```python
from build123d import *

# Parameters (mm, degrees)
BOSS_EXTRU_1_DEPTH      = 1
ESQUISSE2_R             = 1.5
ESQUISSE2_R_2           = 0.5
ENL_V_MAT_EXTRU_1_DEPTH = 18


with BuildPart() as part:
    # Esquisse1 → Boss.-Extru.1 (new body)
    with BuildSketch(Plane.XY):
        with BuildLine():
            Line((-4, 2.530340064), (-4, 15.530340064))
            ThreePointArc((-4, 15.530340064), (0, 19.530340064), (4, 15.530340064))
            Line((4, 15.530340064), (4, 2.530340064))
            Line((4, 2.530340064), (16.535533906, 2.530340064))
            ThreePointArc((16.535533906, 2.530340064), (20.535533906, -1.469659936), (16.535533906, -5.469659936))
            Line((16.535533906, -5.469659936), (4, -5.469659936))
            Line((4, -5.469659936), (4, -19.398592124))
            ThreePointArc((4, -19.398592124), (0, -23.398592124), (-4, -19.398592124))
            Line((-4, -19.398592124), (-4, -5.469659936))
            Line((-4, -5.469659936), (-17.464466094, -5.469659936))
            ThreePointArc((-17.464466094, -5.469659936), (-21.464466094, -1.469659936), (-17.464466094, 2.530340064))
            Line((-17.464466094, 2.530340064), (-4, 2.530340064))
        make_face()
    extrude(amount=BOSS_EXTRU_1_DEPTH)

    # Esquisse2 → Enlèv. mat.-Extru.1 (cut)
    with BuildSketch(Plane.XY.offset(1)):
        with Locations((0, 15.030340064)):
            Circle(ESQUISSE2_R)
        with Locations((16.5, -1.469659936)):
            Circle(ESQUISSE2_R)
        with Locations((0, -17.969659936)):
            Circle(ESQUISSE2_R)
        with Locations((-16.5, -1.469659936)):
            Circle(ESQUISSE2_R)
        with Locations((0, -1.469659936)):
            Circle(ESQUISSE2_R_2)
    extrude(amount=-ENL_V_MAT_EXTRU_1_DEPTH, mode=Mode.SUBTRACT)


solid = part.part
```
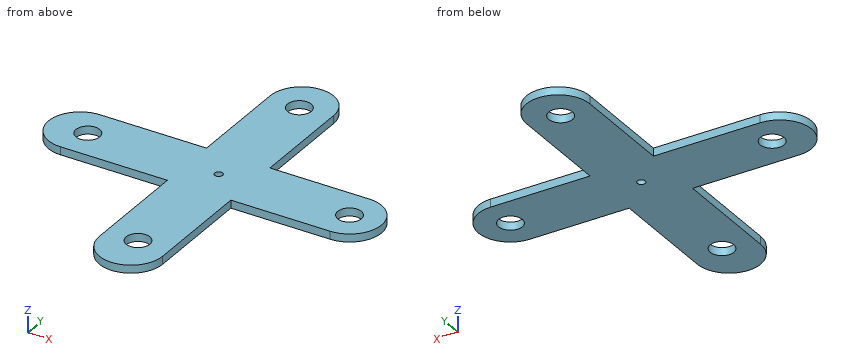
The listing builds one solid part. Answer for the finished solid, in the listing's coordinates (mm). Round coordinates to 2 decimals unless told otherwise and drop trailing zeros. Loops run counter-clockwise (first coordinate to the right, second up) from the corner with the lowest first, then second, coordinate; pieces in that order, holes last.
1) A cutting plane is placed at A-A on x = 0. Determine the outline of the cut face in (y, z).
Outcome:
outline: (-23.4, 0) - (-19.47, 0) - (-19.47, 1) - (-23.4, 1) - close; (-16.47, 0) - (-1.97, 0) - (-1.97, 1) - (-16.47, 1) - close; (-0.97, 0) - (13.53, 0) - (13.53, 1) - (-0.97, 1) - close; (16.53, 0) - (19.53, 0) - (19.53, 1) - (16.53, 1) - close
2) A cutting plane is placed at B-B on x = -16.5. Determine the outline of the cut face in (y, z).
Outcome:
outline: (-5.47, 0) - (-2.97, 0) - (-2.97, 1) - (-5.47, 1) - close; (0.03, 0) - (2.53, 0) - (2.53, 1) - (0.03, 1) - close
3) Given P1, Ø0.5, axis at x = -10, z = 0.5, coming from the -Y side; P2, Ø0.5, axis at x = 9.5, z = 0.5, coming from the +Y side, each flat-ended and moving along its own axis, determine where each tip first touches the part or whether it passes through.
Outcome:
P1: stops at y = -5.47
P2: stops at y = 2.53
4) A cutting plane is placed at D-D on z = 0.4. Determine the outline of the cut face in (x, y).
Outcome:
outline: (-17.46, -5.47) - (-4, -5.47) - (-4, -19.4) arc R4 ccw to (4, -19.4) - (4, -5.47) - (16.54, -5.47) arc R4 ccw to (16.54, 2.53) - (4, 2.53) - (4, 15.53) arc R4 ccw to (-4, 15.53) - (-4, 2.53) - (-17.46, 2.53) arc R4 ccw to start; hole circle Ø3 at (-16.5, -1.47); hole circle Ø3 at (0, -17.97); hole circle Ø3 at (0, 15.03); hole circle Ø1 at (0, -1.47); hole circle Ø3 at (16.5, -1.47)
5) Consider line 1 (Y direction, x = 0, z = 0.85); line 2 (Y direction, x = 16.5, z = 0.45); line 3 (Y direction, x = -10, z = 0.35). Determine where each line is inside the solid, lowest interval first.
Outcome:
line 1: y = -23.4 to -19.47, -16.47 to -1.97, -0.97 to 13.53, 16.53 to 19.53
line 2: y = -5.47 to -2.97, 0.03 to 2.53
line 3: y = -5.47 to 2.53
6) A cutting plane is placed at C-C on y = 14.5. Determine the outline of the cut face in (x, z).
Outcome:
outline: (-4, 0) - (-1.4, 0) - (-1.4, 1) - (-4, 1) - close; (1.4, 0) - (4, 0) - (4, 1) - (1.4, 1) - close
